Answer from the drawing. Dimensions are ordinates in mm from the lowest x, y and z of the part. A direction names the side the tool comes from. Give positions to 0.01 mm unless a question says otherwise; leave off trailing zeros. Write each loop counter-clockwise with the first axis right and the second up, starting at its lowest first coordinate (ties: lowest second). Pieces come first, ordered by that corner, then holes. Notation, with made-up numbers: (37, -38.5) -> (68, -38.5) arc R21 cw to (68, -3.5) -> close; hole circle Ø8 at (9, 15). An arc over 180 degrees is marked (long way). Put each result on its own line as item: value. Start each with the question number.
1) A cutting plane is placed at D-D (z = 48.5). Write down the section's boundary in (x, y), then the cut area to 3 significant figures.
2) A cutting plane is placed at C-C (x = 60). Write down the section's boundary in (y, z).
3) Find the intervals of material crossed by line 1 along Z through (x, y) = (101.5, 44.45); line 2 along Y through (x, z) = (32, 46); line 3 along Y through (x, z) = (100, 16), in increasing order. Write a range as from..to.
4) Flat-ended cylindrical pins translate along their axes: pin 1 Ø1.5 at (y, z) = (31.5, 8.5) entering from -X; pin 2 Ø6 at (x, y) = (61.5, 43) entering from -Z; pin 3 Ø8 at (x, z) = (43.5, 61) entering from -Y. Find the tip coordinate at first contact, or state that the pin passes through.
5) A cutting plane is placed at B-B (y = 41). Write down the section's boundary in (x, z), then the cut area to 3 significant figures.
6) A cutting plane is placed at A-A (z = 12.7). Write down the section's boundary in (x, y), then the cut area to 3 significant figures.
7) For the marked faces 1 and 2, determine the directions among +Z, -Z, +X, -X, +Y, -Y from which every point of the face is accessible in a straight line to the end or side of a thin tool.
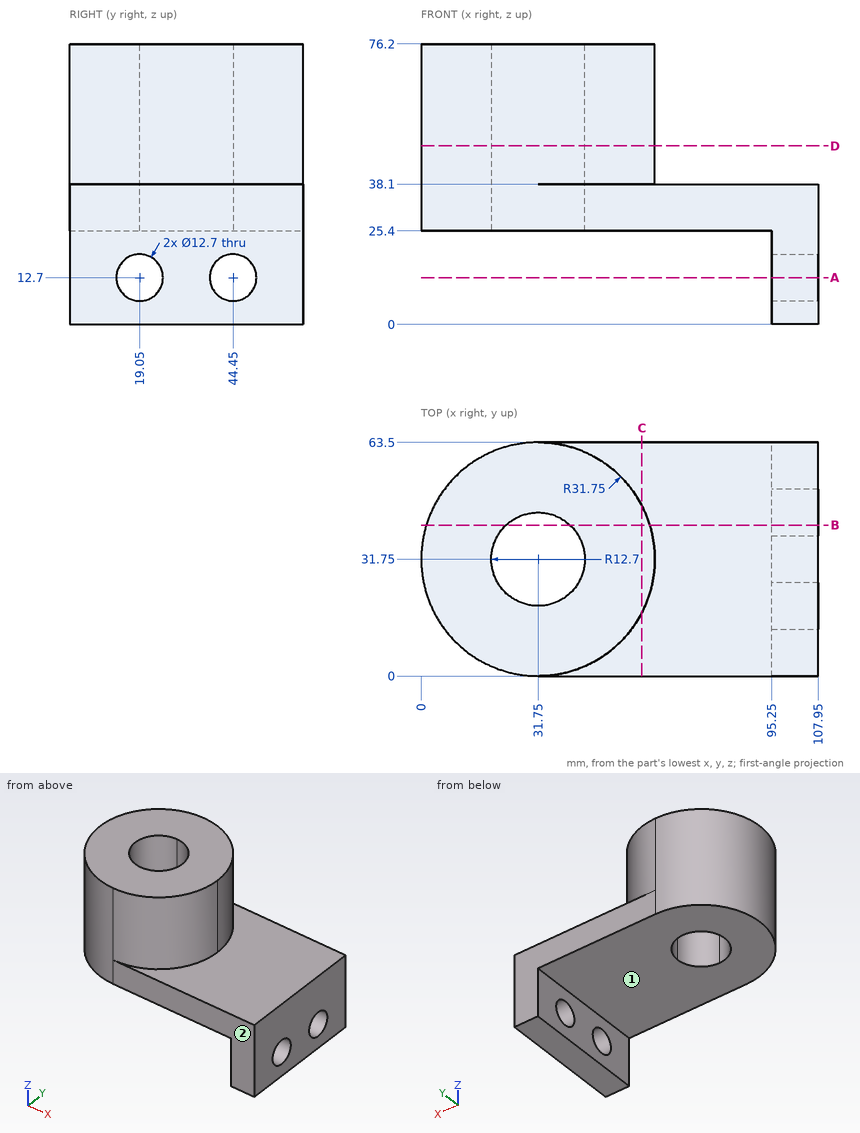
Reply:
1. outline: (31.75, 0) arc R31.75 ccw to (63.5, 31.75) arc R31.75 ccw to (31.75, 63.5) arc R31.75 ccw to start; hole circle Ø25.4 at (31.75, 31.75)
1. area: 2,660 mm2
2. outline: (0, 25.4) -> (63.5, 25.4) -> (63.5, 38.1) -> (46.24, 38.1) -> (46.24, 76.2) -> (17.26, 76.2) -> (17.26, 38.1) -> (0, 38.1) -> close
3. line 1: z = 0..6.35, 19.05..38.1
3. line 2: y = 0..19.05, 44.45..63.5
3. line 3: y = 0..13.62, 24.48..39.02, 49.88..63.5
4. pin 1: stops at x = 95.25
4. pin 2: stops at z = 25.4
4. pin 3: stops at y = 0.96
5. outline: (1.38, 25.4) -> (23.05, 25.4) -> (23.05, 76.2) -> (1.38, 76.2) -> close; (40.45, 25.4) -> (95.25, 25.4) -> (95.25, 18.03) -> (107.95, 18.03) -> (107.95, 38.1) -> (62.12, 38.1) -> (62.12, 76.2) -> (40.45, 76.2) -> close; (95.25, 0) -> (107.95, 0) -> (107.95, 7.37) -> (95.25, 7.37) -> close
5. area: 2,970 mm2
6. outline: (95.25, 0) -> (107.95, 0) -> (107.95, 12.7) -> (95.25, 12.7) -> close; (95.25, 25.4) -> (107.95, 25.4) -> (107.95, 38.1) -> (95.25, 38.1) -> close; (95.25, 50.8) -> (107.95, 50.8) -> (107.95, 63.5) -> (95.25, 63.5) -> close
6. area: 484 mm2
7. face 1: -Z, -X, +Y, -Y
7. face 2: +Z, -Z, +X, -X, -Y
